Design review of the part built by this model. Coordinates are the model's own, in mm. A direction names the side the tool comes from. Round coordinates to 2 decimals unless told otherwise and drop trailing zeros. Loops run counter-clockwise (first coordinate to the right, second up) from the corner with the lowest first, then second, coordinate; pieces in that order, holes last. Notation, with made-up numbers: M -31,64.25 L -15,64.25 A22 ccw -15,73.25 Z; hole C 70.5,-6.75 d8. An arc over 180 degrees is marked long. Use a Markdown table: item, result.
Autodesk Inventor part; units mm, degrees
ref_plane "Work Plane1" through (0, 2.25, -45.5) normal (0, 1, 0) x (-1, 0, 0)
ref_plane "YZ Plane" through (0, 0, 0) normal (1, 0, 0) x (0, 1, 0)
ref_plane "XY Plane" through (0, 0, 0) normal (0, 0, 1) x (1, 0, 0)
sketch "Sketch1" plane through (0, 0, 0) normal (0, 1, 0) x (-1, 0, 0)
  line L0 (0, 9.9065) -> (0, -47)
  line L1 (0, -47) -> (2.25, -47)
  line L2 (2.25, -47) -> (2.25, -44)
  line L3 (2.25, -44) -> (3.175, -44)
  line L4 (3.175, -44) -> (3.175, -10.2)
  line L5 (3.175, -10.2) -> (1.5, -10.2)
  line L6 (1.5, -10.2) -> (1.5, -1)
  line L7 (1.5, -1) -> (1.1, -1)
  line L8 (1.1, -1) -> (1.1, -0.6)
  line L9 (1.1, -0.6) -> (1.5, -0.6)
  line L10 (1.5, -0.6) -> (1.5, 0)
  line L11 (1.5, 0) -> (0, 0)
  dimension "d0" = 33.8
  dimension "d1" = 3
  dimension "d2" = 10.2
  dimension "d3" = 4.5
  dimension "d4" = 6.35
  dimension "d5" = 3
  dimension "d6" = 0.4
  dimension "d7" = 2.2
  dimension "d29" = 1
revolve "Revolution1" add sketch "Sketch1" angle 360 about axis through (0, 0, 9.9065) along (0, 0, -1)
thread "Thread1"
ref_plane "Work Plane1" through (0, 2.25, -45.5) normal (0, 1, 0) x (-1, 0, 0)
sketch "Sketch2" plane through (0, 2.25, -45.5) normal (0, 1, 0) x (-1, 0, 0)
  line L0 (-2.25, -1.5) -> (2.25, -1.5)
  line L1 (0, -1.5) -> (0, 45.5) construction
  point P0 (0, 0)
  dimension "d12" = 1.5
hole "Hole1" at (0, 2.25, -45.5) direction (0, -1, 0) diameter 1.5 end through all
hole "Hole2" at (0, 0, -47) direction (0, 0, 1) diameter 3.1 depth 9 tip angle 118
properties part number "igus_6.35x2.54_screw"
1. The part is to be moulded in two halves that separate along Z. For faces 5 (the face through (1.5, -0.07, -0.3)), 6 (the face through (0.665, -1.809, -45.154)), 7 (the face through (-1.4, -2.1, -44)), say which applies: pulls with the +Z half, pulls with the -Z half, needs draft (parallel to the pull), parting line crosses it, or undercut.
Check values:
| item | result |
|---|---|
| face 5 | needs draft |
| face 6 | undercut |
| face 7 | pulls with the -Z half |
2. Machinability: for faces 1 (the face through (0, 0, 0)), 2 (the face through (-1.05, -0.33, -0.8)), 3 (the face through (-0.07, -1.55, -42.44)), 4 (the face through (1.5, -0.07, -5.54)), which of the approach directions +Z, -Z, +X, -X, +Y, -Y give a long, thin tool a straight path to every point of the face, cutting with its end or side? Answer none if there is none.
Check values:
| item | result |
|---|---|
| face 1 | +Z, +X, -X, +Y, -Y |
| face 2 | none |
| face 3 | -Z |
| face 4 | +Z |
3. Take a section at B-B on z = -25. Give the boundary of the cut face in (x, y) (3 decimals).
Check values:
| item | result |
|---|---|
| outline | C 0,0 d6.35 |
4. Take a section at C-C on x = 2.75. Give the boundary of the cut face in (y, z), and give its area (3 significant figures).
Check values:
| item | result |
|---|---|
| outline | M -1.59,-44 L 1.59,-44 L 1.59,-10.2 L -1.59,-10.2 Z |
| area | 107 mm² |
5. Wall thickness on line 1 along X through (y, z) = (1.8, -45.5); line 2 along Z through (x, y) = (0, -2); line 3 along X through (y, z) = (0.25, -10.5): over which ranges is each line inside the solid? List them lowest first. Write a range as from..to.
Check values:
| item | result |
|---|---|
| line 1 | x = -1.35..-0.75, 0.75..1.35 |
| line 2 | z = -47..-46.25, -44.75..-10.2 |
| line 3 | x = -3.17..3.17 |
6. Insertion check: pin 1 (1.5 mm diameter, centred on x = -1, z = -40.5, fed in from -Y); pin 2 (1.5 mm diameter, centred on x = 0.5, y = -0.5, fed in from -Z); pin 3 (3.5 mm diameter, centred on x = 0.5, y = 0, fed in from +Z); pin 4 (2 mm diameter, centred on x = 0, z = -45.5, fed in from +Y). Each pin has a flat end and moves straight along its axis. Give the tip position at first contact, or say it passes through.
Check values:
| item | result |
|---|---|
| pin 1 | stops at y = -3.17 |
| pin 2 | stops at z = -37.94 |
| pin 3 | stops at z = 0 |
| pin 4 | stops at y = 2.25 |
7. Take a section at A-A on z = -45.5. Give the boundary of the cut face in (x, y), and give its area (3 significant figures).
Check values:
| item | result |
|---|---|
| outline | M -0.75,-2.12 L -0.75,-1.36 A1.55 cw -0.75,1.36 L -0.75,2.12 A2.25 ccw Z; M 0.75,-2.12 A2.25 ccw 0.75,2.12 L 0.75,1.36 A1.55 cw 0.75,-1.36 Z |
| area | 6.20 mm² |
